Here's how the part is built. I have some questions about the finished solid (model axes, mm). Give positions to 0.01 mm unless a question says otherwise; leave off trailing zeros. Loops run counter-clockwise (first coordinate to the right, second up) from the corner with the lowest first, then second, coordinate; pieces in that order, holes last.
Q1. If we section it at B-B (y = 7.5): Please give me the cut outline in (x, z).
Q2. If we section it at D-D (x = -1): Please give me the cut outline in (y, z), plus the area to 3 significant figures.
Q3. If we section it at C-C (z = 2.5): Please give me the cut outline in (x, y), plus the area to 3 significant figures.
Q4. We'd pull the mould along Y, two halves only. Please class faces 1 (the face through (5, -33, 7)), 2 (the face through (5, -50, 3)), 3 (the face through (2.67, 0.256, 3.451)): +Y half, -Y half, draft (parallel to the pull), parting line (faces both ways), or undercut.
Q5. Will these pins go through, and if not, where does the flat tip stop? P1, Ø1, axis at x = 27.5, z = 4, coming from the -Y side; P2, Ø2, axis at y = -9, z = 1.5, coming from the -X side; P3, Ø2, axis at y = -39.5, z = 3, coming from the -X side.
Q6. If we section it at A-A (x = 8.5): Please give me the cut outline in (y, z).
Q7. I need wall thicknesses on line 1 (X direction, y = 10.75, z = 3.75); line 2 (X direction, y = 4.5, z = 3.75); line 3 (Y direction, x = 13, z = 3.75). Which ranges of each line are inside material? Lowest first, please.
from build123d import *
from build123d import SkipClean  # not in build123d's __all__

# Parameters (mm, degrees)
F1_DEPTH = 50
F2_R     = 28
F2_R_2   = 10.75
F3_DEPTH = 7


with BuildPart() as f1:
    # F0 (on Front) → F1 (new body)
    with BuildSketch(Plane.XZ):
        with BuildLine():
            Line((-2, 0), (0, 0))
            Line((0, 0), (10, 0))
            Line((10, 0), (12, 0))
            ThreePointArc((12, 0), (5, 7), (-2, 0))
        make_face()
    extrude(amount=F1_DEPTH)

    # F2 (on Top) → F3 (join)
    with BuildSketch(Plane.XY):
        with Locations((5, 10.75)):
            Circle(F2_R)
        with Locations((5, 10.75)):
            Circle(F2_R_2, mode=Mode.SUBTRACT)
    with SkipClean():  # cleaning this boolean's faces spoils the solid; the shape is the same uncleaned
        extrude(amount=F3_DEPTH)


solid = f1.part
Check sheet entries:
1. outline: (-22.81, 0) - (-5.25, 0) - (-5.25, 7) - (-22.81, 7) - close; (15.25, 0) - (32.81, 0) - (32.81, 7) - (15.25, 7) - close
2. outline: (-50, 0) - (1.83, 0) - (1.83, 7) - (-16.6, 7) - (-16.6, 3.61) - (-50, 3.61) - close; (19.67, 0) - (38.1, 0) - (38.1, 7) - (19.67, 7) - close
2. area: 378 mm2
3. outline: (-1.54, -50) - (11.54, -50) - (11.54, -16.48) arc R28 ccw (long way) to (-1.54, -16.48) - close; hole circle Ø21.5 at (5, 10.75)
3. area: 2,530 mm2
4. face 1: draft
4. face 2: -Y half
4. face 3: undercut
5. P1: stops at y = -6.57
5. P2: stops at x = -15.8
5. P3: stops at x = -1.71
6. outline: (-50, 0) - (0.59, 0) - (0.59, 7) - (-17.03, 7) - (-17.03, 6.06) - (-50, 6.06) - close; (20.91, 0) - (38.53, 0) - (38.53, 7) - (20.91, 7) - close
7. line 1: x = -23 to -5.75, 15.75 to 33
7. line 2: x = -22.29 to -3.75, 13.75 to 32.29
7. line 3: y = -16.08 to 3.57, 17.93 to 37.58
